The model under review builds one solid part; all positions refer to its coordinate system, in mm. Round coordinates to 2 decimals unless told otherwise and drop trailing zeros. Write each loop counter-clockwise with the first axis right and the second up, starting at its lowest first coordinate (ties: lowest second). Pieces come first, ordered by that corner, then holes. Notation, with made-up numbers: (-26.75, 87) -> (-14.75, 87) arc R29 cw to (-14.75, 115) -> close; hole circle Ø3 at (71.25, -28.75). An arc over 180 degrees is marked (long way). Return JSON: item names as keys, results as strings. Group by question number.
1. Take a section at C-C, the plane y = 43.5. Write out the cut boundary in (x, z).
2. For line 1 along X through (y, z) = (66, 0.5); line 2 along Y through (x, z) = (-22, 1.15); line 3 along X through (y, z) = (54.5, 1.65), list the stretches that pass through material, from the lowest coordinate up. Write a range as from..to.
3. Take a section at A-A, the plane y = 0. Write out the cut boundary in (x, z).
4. Take a section at B-B, the plane z = 1.5. Give the number of separate pieces and of enclosed holes in the cut face, then the cut area to 3 significant figures.
5. Take a section at D-D, the plane x = -26. Write out the cut boundary in (y, z), then the cut area to 3 significant figures.
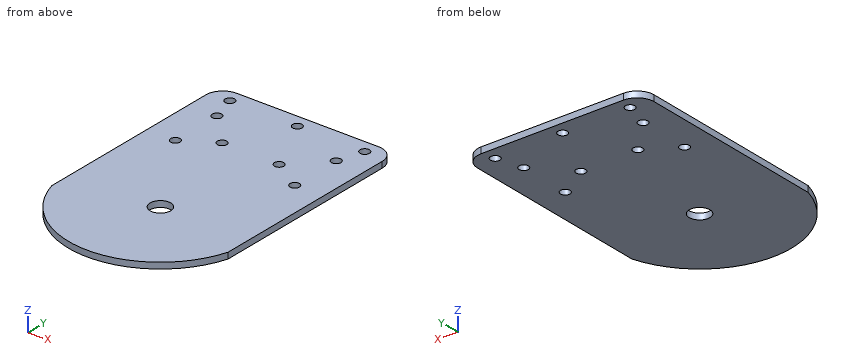
from build123d import *

# Parameters (mm, degrees)
SKETCH1_R             = 4
BOSS_EXTRUDE1_DEPTH   = 2.3368
F_6_CLEARANCE_HOLE1_D = 3.6576
FILLET1_R             = 6.6


with BuildPart() as part:
    # Sketch1 → Boss-Extrude1 (new body)
    with BuildSketch(Plane.XY):
        with BuildLine():
            Line((34, 71), (-34, 71))
            Line((-34, 71), (-34, -9.856977224))
            ThreePointArc((-34, -9.856977224), (0, -35.4), (34, -9.856977224))
            Line((34, -9.856977224), (34, 71))
        make_face()
        Circle(SKETCH1_R, mode=Mode.SUBTRACT)
    extrude(amount=BOSS_EXTRUDE1_DEPTH)

    # #6 Clearance Hole1 (through all)
    with Locations(Plane.XY.offset(2.3368)):
        with Locations((0, 66), (11, 43.5), (23, 36), (23, 56), (26, 66), (-23, 36), (-11, 43.5), (-23, 56), (-26, 66)):
            Hole(F_6_CLEARANCE_HOLE1_D / 2)

    # Fillet1
    fillet1_edges = [part.edges().sort_by_distance(p)[0] for p in [
        (-34, 71, 1.1684),
        (34, 71, 1.1684),
    ]]
    fillet(fillet1_edges, radius=FILLET1_R)


solid = part.part
Output:
{
 "1": {"outline": "(-34, 0) -> (-12.83, 0) -> (-12.83, 2.34) -> (-34, 2.34) -> close; (-9.17, 0) -> (9.17, 0) -> (9.17, 2.34) -> (-9.17, 2.34) -> close; (12.83, 0) -> (34, 0) -> (34, 2.34) -> (12.83, 2.34) -> close"},
 "2": {"line 1": "x = -33.8..-27.83, -24.17..-1.83, 1.83..24.17, 27.83..33.8", "line 2": "y = -27.73..34.47, 37.53..54.47, 57.53..71", "line 3": "x = -34..-24.05, -21.95..21.95, 24.05..34"},
 "3": {"outline": "(-34, 0) -> (-4, 0) -> (-4, 2.34) -> (-34, 2.34) -> close; (4, 0) -> (34, 0) -> (34, 2.34) -> (4, 2.34) -> close"},
 "4": {"separate pieces": "1", "enclosed holes": "10", "area": "6,610 mm^2"},
 "5": {"outline": "(-24.02, 0) -> (64.17, 0) -> (64.17, 2.34) -> (-24.02, 2.34) -> close; (67.83, 0) -> (71, 0) -> (71, 2.34) -> (67.83, 2.34) -> close", "area": "214 mm^2"}
}
